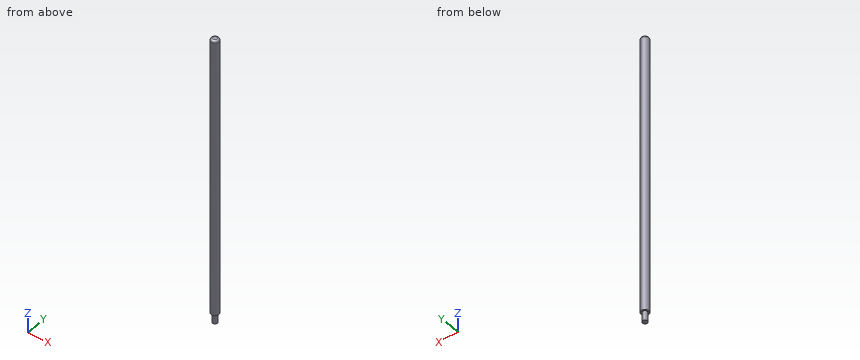
Autodesk Inventor part; units mm, degrees
ref_plane "YZ Plane" through (0, 0, 0) normal (1, 0, 0) x (0, 1, 0)
ref_plane "XZ Plane" through (0, 0, 0) normal (0, 1, 0) x (-1, 0, 0)
ref_plane "XY Plane" through (0, 0, 0) normal (0, 0, 1) x (1, 0, 0)
sketch "Sketch1" plane through (0, 0, 0) normal (0, 0, 1) x (1, 0, 0)
  circle A0 centre (0, 0) radius 4
  dimension "d0" = 8
extrude "Extrusion1" add sketch "Sketch1" along normal mid plane 300
fillet "Fillet1" radius 2 2 edges at (-4, 0, 150) (-4, 0, -150)
thread "Thread1"
sketch "Sketch2" plane through (0, 0, -150) normal (0, 0, -1) x (-1, 0, 0)
  circle A0 centre (0, 0) radius 2 construction
  circle A1 centre (0, 0) radius 4.5
  circle A2 centre (0, 0) radius 4 construction
  circle A3 centre (0, 0) radius 2.5
  dimension "d6" = 0.5
  dimension "d7" = 5
extrude "Extrusion2" cut sketch "Sketch2" against normal blind 10
properties part number "Z Akse gevindstang" material "Aluminum 6061"
CAD build for the part. Positions are in the model's coordinates, mm. Round coordinates to 2 decimals unless told otherwise and drop trailing zeros. Loops run counter-clockwise (first coordinate to the right, second up) from the corner with the lowest first, then second, coordinate; pieces in that order, holes last. Notation, with made-up numbers: M -37.75,-1 L -24.75,-1 A30 cw -24.75,31 Z; hole C 80.25,85.5 d7. An arc over 180 degrees is marked long. One line per question, with ' | ' between items. Start each with the question number.
Item 1: Pin check, flat tips, straight feed: pin 1 Ø2 at (x, z) = (2.5, 29.5) entering from +Y; pin 2 Ø3 at (x, y) = (3, 3) entering from +Z; pin 3 Ø3 at (x, z) = (1.5, -69.5) entering from -Y; pin 4 Ø3 at (y, z) = (-3, 25.5) entering from +X. Stop position of each tip, or through.
Item 2: Cut at A-A, the plane z = 25.5. Write the cut outline in (x, y).
Item 3: Wall check: line 1 (Z direction, x = 2, y = 0.75); line 2 (X direction, y = 0.5, z = 41); line 3 (X direction, y = 0.75, z = -41.5). Give the ranges that are in metal, low to high.
Responses:
1) pin 1: stops at y = 3.71 | pin 2: stops at z = 149.86 | pin 3: stops at y = -4 | pin 4: stops at x = 3.71
2) outline: C 0,0 d8
3) line 1: z = -150 to 150 | line 2: x = -3.97 to 3.97 | line 3: x = -3.93 to 3.93
